```python
from build123d import *

# Parameters (mm, degrees)
CROQUIS1_W              = 10
CROQUIS1_H              = 90
SALIENTE_EXTRUIR1_DEPTH = 7
CROQUIS2_R              = 2.5
CORTAR_EXTRUIR1_DEPTH   = 46.814844756
REDONDEO1_R             = 2


with BuildPart() as part:
    # Croquis1 → Saliente-Extruir1 (new body)
    with BuildSketch(Plane.XY):
        Rectangle(CROQUIS1_W, CROQUIS1_H)
    extrude(amount=SALIENTE_EXTRUIR1_DEPTH)

    # Croquis2 → Cortar-Extruir1 (cut, through all)
    with BuildSketch(Plane.XY.offset(7)):
        with Locations((0, -35)):
            Circle(CROQUIS2_R)
        with Locations((0, -15)):
            Circle(CROQUIS2_R)
    extrude(amount=-CORTAR_EXTRUIR1_DEPTH, mode=Mode.SUBTRACT)

    # Redondeo1
    redondeo1_edges = [part.edges().sort_by_distance(p)[0] for p in [
        (-5, 45, 3.5),
        (5, 45, 3.5),
        (5, -45, 3.5),
        (-5, -45, 3.5),
    ]]
    fillet(redondeo1_edges, radius=REDONDEO1_R)


solid = part.part
```
Read the model definition and answer for the solid it produces. Units are mm, in the model's axes. Give positions to 0.01 mm unless a question says otherwise; leave off trailing zeros. Write each loop counter-clockwise with the first axis right and the second up, starting at its lowest first coordinate (ties: lowest second). Pieces come first, ordered by that corner, then holes. Notation, with made-up numbers: M 53.5,11 L 80.5,11 A29 ccw 80.5,34 Z; hole C -9,1 d4. An arc over 180 degrees is marked long. Put each result on its own line as item: value. Start each with the question number.
1. For a pull along Y with two mould halves and no side action, classify faces 1 (the flat face through (0, 1, 0)), 2 (the flat face through (0, 45, 3)), 3 (the cylindrical face through (-0.54, -17.44, 3.55)) as released by +Y, released by -Y, zero draft, split by the parting line, or undercut.
2. The part is cut by section A-A, the plane y = -35. Give the vertices of the cut face in (x, z), and give its area (3 significant figures).
3. Consider line 1 along Y through (x, z) = (0, 5.75); line 2 along Y through (x, z) = (1.5, 3.75); line 3 along X through (y, z) = (-36, 2.75). Determine where each line is inside the solid, lowest interval first.
4. The part is cut by section B-B, the plane x = 0. Give the vertices of the cut face in (y, z).
5. Each of these flat-tipped pins is pushed along its axis until it touches: pin 1 Ø1.5 at (x, y) = (-1, 9) entering from -Z; pin 2 Ø1.5 at (x, z) = (-4, 3.5) entering from +Y; pin 3 Ø4 at (x, y) = (0, -15) entering from -Z. Where does it stop, or does it pass through?
6. The part is cut by section C-C, the plane z = 2. Give the vertices of the cut face in (x, y), and give its area (3 significant figures).
Final values:
1. face 1: zero draft
1. face 2: released by +Y
1. face 3: undercut
2. outline: M -5,0 L -2.5,0 L -2.5,7 L -5,7 Z; M 2.5,0 L 5,0 L 5,7 L 2.5,7 Z
2. area: 35.0 mm²
3. line 1: y = -45 to -37.5, -32.5 to -17.5, -12.5 to 45
3. line 2: y = -45 to -37, -33 to -17, -13 to 45
3. line 3: x = -5 to -2.29, 2.29 to 5
4. outline: M -45,0 L -37.5,0 L -37.5,7 L -45,7 Z; M -32.5,0 L -17.5,0 L -17.5,7 L -32.5,7 Z; M -12.5,0 L 45,0 L 45,7 L -12.5,7 Z
5. pin 1: stops at z = 0
5. pin 2: stops at y = 44.98
5. pin 3: passes through
6. outline: M -5,-43 A2 ccw -3,-45 L 3,-45 A2 ccw 5,-43 L 5,43 A2 ccw 3,45 L -3,45 A2 ccw -5,43 Z; hole C 0,-35 d5; hole C 0,-15 d5
6. area: 857 mm²
